Can you work these out from the model? Positions are in its coordinate system, mm. Round coordinates to 2 decimals unless told otherwise and drop trailing zeros. Loops run counter-clockwise (first coordinate to the right, second up) from the corner with the lowest first, then second, coordinate; pieces in that order, holes last. Notation, with made-up numbers: (11.25, 81.5) - (21.25, 81.5) arc R21 ccw to (21.25, 112.5) - close; hole circle Ø8 at (80.25, 60). An arc over 180 degrees is marked (long way). Answer as CSV lines item,"result".
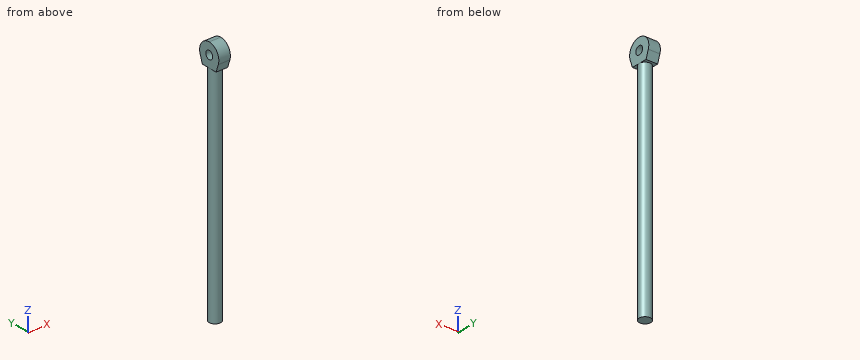
```python
from build123d import *

# Parameters (mm, degrees)
SKETCH1_R           = 17.5
BOSS_EXTRUDE1_DEPTH = 679
BOSS_EXTRUDE3_DEPTH = 17.5
SKETCH5_R           = 12.5
CUT_EXTRUDE1_DEPTH  = 35


with BuildPart() as part:
    # Sketch1 → Boss-Extrude1 (new body)
    with BuildSketch(Plane.XY):
        Circle(SKETCH1_R)
    extrude(amount=BOSS_EXTRUDE1_DEPTH)

    # Sketch3 → Boss-Extrude3 (add, symmetric)
    with BuildSketch(Plane(origin=(0, 0, 0), x_dir=(0, 0, -1), z_dir=(1, 0, 0))):
        with BuildLine():
            Line((-679, 0), (-749, 0))
            ThreePointArc((-749, 0), (-734.34333678, 28.480671492), (-702.648648649, 33.108108108))
            Line((-702.648648649, 33.108108108), (-679, 25))
            Line((-679, 25), (-679, 0))
        make_face()
    boss_extrude3 = extrude(amount=BOSS_EXTRUDE3_DEPTH, both=True)

    # Mirror3: Boss-Extrude3 across plane
    add(boss_extrude3.mirror(Plane(origin=(17.5, 0, 679), x_dir=(0, 0, 1), z_dir=(0, 1, 0))))

    # Sketch5 → Cut-Extrude1 (cut)
    with BuildSketch(Plane(origin=(17.5, 0, 0), x_dir=(0, 0, -1), z_dir=(1, 0, 0))):
        with Locations((-714, 0)):
            Circle(SKETCH5_R)
    extrude(amount=-CUT_EXTRUDE1_DEPTH, mode=Mode.SUBTRACT)


solid = part.part
```
Q1. Imagine slicing it at C-C (z = 418). Write out the boundary of the cut face in (x, y), then the cut area to 3 significant figures.
Checks:
outline,"circle Ø35 at (0, 0)"
area,"962 mm²"
Q2. Imagine slicing it at A-A (x = 0). Write out the boundary of the cut face in (y, z), then the cut area to 3 significant figures.
Checks:
outline,"(-33.11, 702.65) - (-25, 679) - (-17.5, 679) - (-17.5, 0) - (17.5, 0) - (17.5, 679) - (25, 679) - (33.11, 702.65) arc R35 ccw (long way) to start; hole circle Ø25 at (0, 714)"
area,"27,400 mm²"
Q3. I'm going to push flat-ended pins straight in: pin 1 Ø3 at (y, z) = (16, 91.5) entering from +X; pin 2 Ø12 at (x, y) = (-2, -14) entering from +Z; pin 3 Ø4 at (x, z) = (-13, 266) entering from -Y. Where does each tip first touch, or does it pass through?
Checks:
pin 1,"x = 9.8"
pin 2,"z = 748.07"
pin 3,"y = -13.61"
Q4. If I drill on line 1 along Z through (x, y) = (-16, 1.5); line 2 along Y through (x, z) = (0, 714); line 3 along X through (y, z) = (1.5, 453.5), over which ranges is the centre line in solid material (lowest first)? Write a range as [from, to].
Checks:
line 1,"[0, 701.59], [726.41, 748.97]"
line 2,"[-35, -12.5], [12.5, 35]"
line 3,"[-17.44, 17.44]"
Q5. Imagine slicing it at B-B (z = 714). Write out the boundary of the cut face in (x, y).
Checks:
outline,"(-17.5, -35) - (17.5, -35) - (17.5, -12.5) - (-17.5, -12.5) - close; (-17.5, 12.5) - (17.5, 12.5) - (17.5, 35) - (-17.5, 35) - close"
